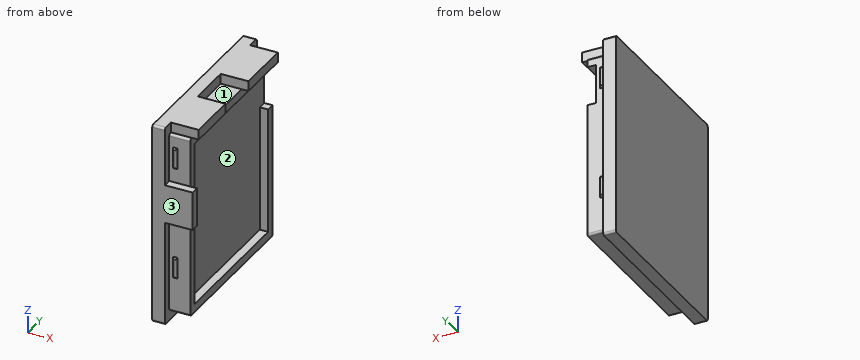
Autodesk Inventor part; units mm, degrees
ref_plane "YZ Plane" through (0, 0, 0) normal (1, 0, 0) x (0, 1, 0)
ref_plane "XZ Plane" through (0, 0, 0) normal (0, 1, 0) x (-1, 0, 0)
ref_plane "XY Plane" through (0, 0, 0) normal (0, 0, 1) x (1, 0, 0)
sketch "Sketch1" plane through (0, 0, 0) normal (1, 0, 0) x (0, 1, 0)
  line L0 (9.8886, 10.374) -> (-32.1114, 10.374)
  line L1 (-32.1114, 10.374) -> (-32.1114, -37.736)
  line L2 (-32.1114, -37.736) -> (9.8886, -37.736)
  line L3 (9.8886, -37.736) -> (9.8886, 10.374)
  point P0 (0, 0)
  dimension "d0" = 42
  dimension "d1" = 48.11
extrude "Extrusion1" add sketch "Sketch1" along normal blind 3
sketch "Sketch2" plane through (3, 0, 0) normal (1, 0, 0) x (0, 0, -1)
  line L0 (-7.974, 7.4886) -> (35.336, 7.4886)
  line L1 (35.336, 7.4886) -> (35.336, -30.1114)
  line L2 (35.336, -30.1114) -> (-7.974, -30.1114)
  line L3 (-7.974, -30.1114) -> (-7.974, 7.4886)
  line L4 (37.736, 9.8886) -> (-10.374, 9.8886)
  line L5 (-10.374, 9.8886) -> (-10.374, -32.1114)
  line L6 (-10.374, -32.1114) -> (37.736, -32.1114)
  point P0 (0, 0)
  dimension "d4" = 43.31
  dimension "d6" = 2.4
  dimension "d7" = 2.4
  dimension "d20" = 2
extrude "Extrusion2" add sketch "Sketch2" along normal blind 3
fillet "Fillet1" radius 0.5 4 edges at (1.5, 9.8886, 10.374) (1.5, 9.8886, -37.736) (1.5, -32.1114, 10.374) (1.5, -32.1114, -37.736)
sketch "Sketch3" plane through (3, 0, 0) normal (1, 0, 0) x (0, 0, -1)
  line L0 (-10.374, 9.3886) -> (-10.374, -31.6114)
  line L1 (-7.974, -30.1114) -> (-7.974, 7.4886)
  line L2 (-10.374, -29.3114) -> (-7.974, -29.3114)
  line L3 (-7.974, -29.3114) -> (-7.974, -17.1114)
  line L4 (-7.974, -17.1114) -> (-10.374, -17.1114)
  line L5 (-10.374, -17.1114) -> (-10.374, -29.3114)
  line L6 (-9.874, -32.1114) -> (37.236, -32.1114)
  point P0 (0, 0)
  point P1 (-7.974, -29.6114)
  point P2 (-7.974, 6.9886)
  point P3 (-7.974, -29.3114)
  dimension "d12" = 12.2
  dimension "d13" = 2.8
extrude "PowerSocket" add sketch "Sketch3" along normal blind 6.6
sketch "Sketch5" plane through (3, 0, 0) normal (1, 0, 0) x (0, 0, -1)
  line L0 (-10.374, 9.3886) -> (-10.374, -17.1114)
  line L1 (-7.974, -17.1114) -> (-7.974, 7.4886)
  line L2 (-10.374, -6.6114) -> (-7.974, -6.6114)
  line L3 (-7.974, -6.6114) -> (-7.974, 6.7886)
  line L4 (-7.974, 6.7886) -> (-10.374, 6.7886)
  line L5 (-10.374, 6.7886) -> (-10.374, -6.6114)
  line L6 (-7.974, -17.1114) -> (-10.374, -17.1114)
  line L7 (35.336, 7.4886) -> (-7.974, 7.4886)
  line L8 (37.236, 9.8886) -> (-9.874, 9.8886)
  point P0 (0, 0)
  point P1 (-10.374, 6.7886)
  point P2 (-7.974, -6.6114)
  dimension "d21" = 13.4
  dimension "d75" = 3.1
extrude "RJ-12" add sketch "Sketch5" along normal blind 6.6 contours L4 L1 L2 L0
sketch "Sketch6" plane through (3, 0, 0) normal (1, 0, 0) x (0, 0, -1)
  line L0 (-9.874, -32.1114) -> (37.236, -32.1114)
  line L1 (-7.974, -30.1114) -> (35.336, -30.1114)
  line L2 (12.726, -32.1114) -> (3.526, -32.1114)
  line L3 (3.526, -32.1114) -> (3.526, -30.1114)
  line L4 (3.526, -30.1114) -> (12.726, -30.1114)
  line L5 (12.726, -30.1114) -> (12.726, -32.1114)
  line L6 (-10.374, -29.3114) -> (-10.374, -31.6114)
  point P0 (0, 0)
  dimension "d25" = 9.2
  dimension "d26" = 13.9
extrude "USB-C" add sketch "Sketch6" along normal blind 6.6
sketch "Sketch7" plane through (6, 0, 0) normal (1, 0, 0) x (0, 0, -1)
  line L0 (35.336, 7.4886) -> (-7.974, 7.4886)
  line L1 (-7.974, 7.4886) -> (-5.974, 7.4886)
  line L2 (-5.974, 7.4886) -> (-5.974, -30.1114)
  line L3 (-7.974, -30.1114) -> (3.526, -30.1114)
  line L4 (-5.974, -30.1114) -> (-7.974, -30.1114)
  line L5 (-10.374, -29.3114) -> (-10.374, -31.6114)
  line L6 (-7.974, 7.4886) -> (-7.974, -17.1114)
  line L7 (-7.974, -30.1114) -> (-7.974, 7.4886)
  line L8 (35.336, -30.1114) -> (12.726, -30.1114)
  line L9 (-5.974, -30.1114) -> (35.336, -30.1114)
  line L10 (35.336, -30.1114) -> (35.336, -28.1114)
  line L11 (35.336, 7.4886) -> (35.336, -30.1114)
  line L12 (35.336, -28.1114) -> (-5.974, -28.1114)
  line L13 (35.336, -28.1114) -> (35.336, 7.4886)
  line L14 (35.336, 7.4886) -> (33.336, 7.4886)
  line L15 (33.336, 7.4886) -> (33.336, -28.1114)
  line L16 (33.336, 7.4886) -> (3.336, 7.4886)
  line L17 (3.336, 7.4886) -> (3.336, 5.4886)
  line L18 (3.336, 5.4886) -> (33.336, 5.4886)
  point P0 (0, 0)
  point P1 (-7.974, 6.7886)
  point P2 (-7.974, 6.6886)
  dimension "d29" = 2
  dimension "d30" = 2
  dimension "d31" = 2
  dimension "d32" = 2
  dimension "d33" = 30
  dimension "d34" = 2
extrude "Extrusion7" add sketch "Sketch7" along normal blind 2 contours L11 L12 L15 L0 | L15 L18 L17 L0 | L10 L8 L9 L3 L2 L12 | L2 L3 L7 L6 L0
sketch "Sketch8" plane through (3, -30.1114, -3.526) normal (0, -1, 0) x (1, 0, 0)
  line L0 (2, 8.5) -> (1, 8.5)
  line L1 (1, 8.5) -> (1, 3.5)
  line L2 (1, 3.5) -> (2, 3.5)
  line L3 (2, 3.5) -> (2, 8.5)
  line L4 (0, 11.5) -> (5, 11.5)
  line L5 (5, 11.5) -> (5, 0)
  line L6 (0, 13.4) -> (0, 0)
  point P0 (-3, 3.526)
  point P1 (2, 6)
  dimension "d37" = 1
  dimension "d38" = 5
  dimension "d39" = 5.5
  dimension "d60" = 1
extrude "Extrusion8" add sketch "Sketch8" along normal blind 0.5
fillet "Fillet3" radius 0.5 4 edges at (5, -30.6114, 2.474) (4, -30.6114, 2.474) (4.5, -30.6114, 4.974) (4.5, -30.6114, -0.026)
sketch "Sketch9" plane through (3, -30.1114, -35.336) normal (0, -1, 0) x (1, 0, 0)
  line L0 (2, 13.5) -> (1, 13.5)
  line L1 (1, 13.5) -> (1, 8.5)
  line L2 (1, 8.5) -> (2, 8.5)
  line L3 (2, 8.5) -> (2, 13.5)
  line L4 (5, 22.61) -> (5, 0)
  line L5 (0, 0) -> (5, 0)
  line L6 (0, 22.61) -> (0, -1.9)
  point P0 (-3, 35.336)
  point P1 (2, 11)
  dimension "d44" = 1
  dimension "d45" = 5
  dimension "d47" = 11
  dimension "d59" = 1
extrude "Extrusion9" add sketch "Sketch9" along normal blind 0.5
fillet "Fillet4" radius 0.5 4 edges at (5, -30.6114, -24.336) (4, -30.6114, -24.336) (4.5, -30.6114, -21.836) (4.5, -30.6114, -26.836)
sketch "Sketch10" plane through (3, 7.4886, 7.974) normal (0, 1, 0) x (1, 0, 0)
  line L0 (2, 34.81) -> (1, 34.81)
  line L1 (1, 34.81) -> (1, 29.81)
  line L2 (1, 29.81) -> (2, 29.81)
  line L3 (2, 29.81) -> (2, 34.81)
  line L4 (5, 43.31) -> (5, 11.31)
  line L5 (0, 43.31) -> (5, 43.31)
  line L6 (0, 45.21) -> (0, -1.9)
  point P0 (-3, 7.974)
  point P1 (2, 32.31)
  dimension "d51" = 1
  dimension "d52" = 5
  dimension "d54" = 11
  dimension "d58" = 1
extrude "Extrusion10" add sketch "Sketch10" along normal blind 0.5
fillet "Fillet5" radius 0.5 4 edges at (5, 7.9886, -24.336) (4, 7.9886, -24.336) (4.5, 7.9886, -26.836) (4.5, 7.9886, -21.836)
sketch "Sketch11" plane through (3, 7.4886, 7.974) normal (0, 1, 0) x (1, 0, 0)
  line L0 (2, 8) -> (1, 8)
  line L1 (1, 8) -> (1, 3)
  line L2 (1, 3) -> (2, 3)
  line L3 (2, 3) -> (2, 8)
  line L4 (0, 45.21) -> (0, -1.9)
  line L5 (0, 0) -> (5, 0)
  point P0 (-3, 7.974)
  point P1 (1, 5.5)
  dimension "d61" = 1
  dimension "d62" = 5
  dimension "d63" = 1
  dimension "d64" = 5.5
extrude "Extrusion11" add sketch "Sketch11" along normal blind 0.5
fillet "Fillet6" radius 0.5 4 edges at (5, 7.9886, 2.474) (4, 7.9886, 2.474) (4.5, 7.9886, 4.974) (4.5, 7.9886, -0.026)
fillet "Fillet7" radius 0.5 4 edges at (5.5, -30.1114, -35.336) (5.5, 7.4886, -35.336) (5.5, 7.4886, 7.974) (5.5, -30.1114, 7.974)
properties part number "Enclosure_Bottom"
Could you check a few things on this model? Use its own coordinates, in mm. Face numbers are marked on the shaded views. Give positions to 0.01 mm unless a question says otherwise; leave off trailing zeros. Order: outer loops, then holes, each group sorted by start corner. A loop starts at its lowest first (then second) coordinate and runs counter-clockwise, first axis right, second up.
Q1. If I drill on line 1 along Z through (x, y) = (7.25, -7.5); line 2 along Y through (x, z) = (7.25, 8.5); line 3 along Z through (x, y) = (7.75, -3.5), over which ranges is the centre line in solid material (lowest first)?
Q2. We'd pull the mould along Z, two halves only. Please class the marked faces 1, 2 and 3: +Z half, -Z half, draft (parallel to the pull), parting line (faces both ways), or undercut.
Q3. Suppose I cut it at D-D, the plane y = -10. Write out the boundary of the cut face in (x, z), and give its area (3 significant figures).
Q4. Suppose I cut it at A-A, the plane x = 8.75. Write out the boundary of the cut face in (y, z), and give its area (3 significant figures).
Q5. I'm going to push flat-ended pins straight in: P1, Ø1, axis at x = 7, z = -20.5, coming from the -Y side; P2, Ø10, axis at y = -14.5, z = -15.5, coming from the +X side; P3, Ø1.9, axis at x = 5, z = 9.5, coming from the -Y side. Where does each tip first touch, or does it pass through?
Q6. Suppose I cut it at C-C, the plane y = -20. Write out the boundary of the cut face in (x, z).
Solution:
1. line 1: z = -35.34 to -33.34, 5.97 to 7.97
1. line 2: y = -29.31 to -17.11, -6.61 to 6.79
1. line 3: z = -35.34 to -33.34, 5.97 to 10.37
2. face 1: +Z half
2. face 2: undercut
2. face 3: draft
3. outline: (0, -37.74) - (3, -37.74) - (3, -35.34) - (8, -35.34) - (8, -33.34) - (6, -33.34) - (6, 5.97) - (8, 5.97) - (8, 7.97) - (3, 7.97) - (3, 10.37) - (0, 10.37) - close
3. area: 282 mm2
4. outline: (-32.11, -12.73) - (-30.11, -12.73) - (-30.11, -3.53) - (-32.11, -3.53) - close; (-29.31, 7.97) - (-17.11, 7.97) - (-17.11, 10.37) - (-29.31, 10.37) - close; (-6.61, 7.97) - (6.79, 7.97) - (6.79, 10.37) - (-6.61, 10.37) - close
4. area: 79.8 mm2
5. P1: stops at y = -30.11
5. P2: stops at x = 6
5. P3: stops at y = -29.31
6. outline: (0, -37.74) - (3, -37.74) - (3, -35.34) - (8, -35.34) - (8, -33.34) - (6, -33.34) - (6, 5.97) - (8, 5.97) - (8, 7.97) - (9.6, 7.97) - (9.6, 10.37) - (0, 10.37) - close
